Input: part model. Units: mm. Frame: model coordinates. A direction names the side the tool comes from. Coordinates: 2 decimals unless noted, no trailing zeros. Write each loop counter-clockwise with the first axis right and the second up, starting at its lowest first coordinate (ties: lowest second). Pieces come first, ordered by that corner, then holes. Notation, with made-up numbers: (63, -8) - (112, -8) arc R9 cw to (112, 9) - close; hole circle Ø11 at (37, -20). An arc over 180 degrees is marked (long way). Put each result on its own line as item: value. Start each with the question number.
1. Cut plane C-C, the plane y = -24.5. Return loops of the section in (x, z).
2. Line query: line 1 (Y direction, x = -40, z = 2.15); line 2 (Z direction, x = -21, y = 18); line 3 (Z direction, x = 31, y = 27). Output: solid intervals per line, ascending.
3. Cut plane A-A, the plane x = -7.5. Return loops of the section in (y, z), and give its area (3 significant figures).
4. Pull-direction query (X, two-part tool) for faces 5 (the flat face through (-38, -32.5, 1)), 6 (the cylindrical face through (43.57, 31, 1.52)), 7 (the flat face through (30, 22, 8)); classes: released by +X, released by -X, zero draft, split by the parting line, or undercut.
5. Access query for faces 1 (the flat face through (-1, 12.5, 28)), 2 (the flat face through (-30, -22, 9)), 3 (the flat face through (37, -27, 3)), 4 (the flat face through (-11, 22.5, 24)). Directions: +Z, -Z, +X, -X, +Y, -Y. A direction counts if a zero-diameter tool reaches every point of the face in a straight line with its end or side. Return the directions, or none.
6. Cut plane B-B, the plane y = -10. Return loops of the section in (x, z).
7. Pin query (flat end, axial travel): pin 1 (5 mm diameter, centred on x = 36.5, y = 27, fed in from +Z); pin 2 (1 mm diameter, centred on x = 9.5, y = 22, fed in from -Z); pin 3 (10 mm diameter, centred on x = -21.5, y = -13.5, fed in from -Z); pin 4 (5.5 mm diameter, centred on y = 24, z = 6.5, fed in from -X). Return the tip coordinate at first contact, or that it passes through.
8. Cut plane D-D, the plane y = -16.5. Return loops of the section in (x, z).
from build123d import *

# Parameters (mm, degrees)
SKETCH1_W           = 90
SKETCH1_H           = 65
BOSS_EXTRUDE1_DEPTH = 3
FILLET4_R           = 5
FILLET5_R           = 5
FILLET6_R           = 5
FILLET7_R           = 5
SKETCH4_W           = 90
SKETCH4_H           = 45
BOSS_EXTRUDE2_DEPTH = 26
SKETCH6_W           = 90
SKETCH6_H           = 41
CUT_EXTRUDE2_DEPTH  = 27
SKETCH5_W           = 80
SKETCH5_H           = 25
CUT_EXTRUDE3_DEPTH  = 3
SKETCH7_R           = 2
CUT_EXTRUDE4_DEPTH  = 3
SKETCH8_R           = 2
CUT_EXTRUDE5_DEPTH  = 3
SKETCH10_W          = 60
SKETCH10_H          = 22
CUT_EXTRUDE7_DEPTH  = 12
FILLET9_R           = 5
FILLET10_R          = 5
SKETCH11_W          = 60
SKETCH11_H          = 22
CUT_EXTRUDE8_DEPTH  = 12
FILLET11_R          = 5
FILLET12_R          = 5


with BuildPart() as part:
    # Sketch1 → Boss-Extrude1 (new body)
    with BuildSketch(Plane.XY):
        Rectangle(SKETCH1_W, SKETCH1_H)
    extrude(amount=BOSS_EXTRUDE1_DEPTH)

    # Fillet4
    fillet4_edges = [part.edges().sort_by_distance(p)[0] for p in [
        (-45, -32.5, 1.5),
    ]]
    fillet(fillet4_edges, radius=FILLET4_R)

    # Fillet5
    fillet5_edges = [part.edges().sort_by_distance(p)[0] for p in [
        (45, -32.5, 1.5),
    ]]
    fillet(fillet5_edges, radius=FILLET5_R)

    # Fillet6
    fillet6_edges = [part.edges().sort_by_distance(p)[0] for p in [
        (45, 32.5, 1.5),
    ]]
    fillet(fillet6_edges, radius=FILLET6_R)

    # Fillet7
    fillet7_edges = [part.edges().sort_by_distance(p)[0] for p in [
        (-45, 32.5, 1.5),
    ]]
    fillet(fillet7_edges, radius=FILLET7_R)

    # Sketch4 → Boss-Extrude2 (add)
    with BuildSketch(Plane.XY.offset(3)):
        Rectangle(SKETCH4_W, SKETCH4_H)
    extrude(amount=BOSS_EXTRUDE2_DEPTH)

    # Sketch6 → Cut-Extrude2 (cut)
    with BuildSketch(Plane(origin=(0, 0, 0), x_dir=(-1, 0, 0), z_dir=(0, 0, -1))):
        Rectangle(SKETCH6_W, SKETCH6_H)
    extrude(amount=-CUT_EXTRUDE2_DEPTH, mode=Mode.SUBTRACT)

    # Sketch5 → Cut-Extrude3 (cut)
    with BuildSketch(Plane.XY.offset(29)):
        Rectangle(SKETCH5_W, SKETCH5_H)
    extrude(amount=-CUT_EXTRUDE3_DEPTH, mode=Mode.SUBTRACT)

    # Sketch7 → Cut-Extrude4 (cut)
    with BuildSketch(Plane.XY.offset(3)):
        with Locations((40, -27.5)):
            Circle(SKETCH7_R)
        with Locations((-40, -27.5)):
            Circle(SKETCH7_R)
    extrude(amount=-CUT_EXTRUDE4_DEPTH, mode=Mode.SUBTRACT)

    # Sketch8 → Cut-Extrude5 (cut)
    with BuildSketch(Plane.XY.offset(3)):
        with Locations((-40, 27.5)):
            Circle(SKETCH8_R)
        with Locations((40, 27.5)):
            Circle(SKETCH8_R)
    extrude(amount=-CUT_EXTRUDE5_DEPTH, mode=Mode.SUBTRACT)

    # Sketch10 → Cut-Extrude7 (cut)
    with BuildSketch(Plane.XZ.offset(-20.5)):
        with Locations((0, 11)):
            Rectangle(SKETCH10_W, SKETCH10_H)
    extrude(amount=-CUT_EXTRUDE7_DEPTH, mode=Mode.SUBTRACT)

    # Fillet9
    fillet9_edges = [part.edges().sort_by_distance(p)[0] for p in [
        (-30, 32.5, 1.5),
    ]]
    fillet(fillet9_edges, radius=FILLET9_R)

    # Fillet10
    fillet10_edges = [part.edges().sort_by_distance(p)[0] for p in [
        (30, 32.5, 1.5),
    ]]
    fillet(fillet10_edges, radius=FILLET10_R)

    # Sketch11 → Cut-Extrude8 (cut)
    with BuildSketch(Plane(origin=(0, -20.5, 0), x_dir=(1, 0, 0), z_dir=(0, 1, 0))):
        with Locations((0, -11)):
            Rectangle(SKETCH11_W, SKETCH11_H)
    extrude(amount=-CUT_EXTRUDE8_DEPTH, mode=Mode.SUBTRACT)

    # Fillet11
    fillet11_edges = [part.edges().sort_by_distance(p)[0] for p in [
        (30, -32.5, 1.5),
    ]]
    fillet(fillet11_edges, radius=FILLET11_R)

    # Fillet12
    fillet12_edges = [part.edges().sort_by_distance(p)[0] for p in [
        (-30, -32.5, 1.5),
    ]]
    fillet(fillet12_edges, radius=FILLET12_R)


solid = part.part
Report:
1. outline: (-45, 0) - (-30, 0) - (-30, 3) - (-45, 3) - close; (30, 0) - (45, 0) - (45, 3) - (30, 3) - close
2. line 1: y = -32.5 to -29.5, -25.5 to -20.5, 20.5 to 25.5, 29.5 to 32.5
2. line 2: z = 27 to 29
2. line 3: z = 0 to 3
3. outline: (-22.5, 22) - (-20.5, 22) - (-20.5, 27) - (-12.5, 27) - (-12.5, 29) - (-22.5, 29) - close; (12.5, 27) - (20.5, 27) - (20.5, 22) - (22.5, 22) - (22.5, 29) - (12.5, 29) - close
3. area: 60.0 mm^2
4. face 5: zero draft
4. face 6: released by +X
4. face 7: undercut
5. face 1: +Z, -Z
5. face 2: -Z, +Y, -Y
5. face 3: +Z, +X, -X, -Y
5. face 4: +Z, +X, -X, +Y
6. outline: (-45, 27) - (-40, 27) - (-40, 29) - (-45, 29) - close; (40, 27) - (45, 27) - (45, 29) - (40, 29) - close
7. pin 1: stops at z = 3
7. pin 2: stops at z = 22
7. pin 3: stops at z = 27
7. pin 4: stops at x = -45
8. outline: (-45, 27) - (45, 27) - (45, 29) - (-45, 29) - close
